from build123d import *

# Parameters (mm, degrees)
CYLINDER002_R     = 2.5
CYLINDER002_DEPTH = 18
CYLINDER003_R     = 4.5
CYLINDER003_DEPTH = 5
CYLINDER_R        = 2.5
CYLINDER_DEPTH    = 18
CYLINDER001_R     = 4.5
CYLINDER001_DEPTH = 5
PAD_DEPTH         = 12


with BuildPart() as cilindro002:
    # Cylinder002 → Cylinder002 (new body)
    with BuildSketch(Plane.XY):
        Circle(CYLINDER002_R)
    extrude(amount=CYLINDER002_DEPTH)


with BuildPart() as obj1:
    # Cylinder003 → Cylinder003 (new body)
    with BuildSketch(Plane.XY.offset(18)):
        Circle(CYLINDER003_R)
    extrude(amount=CYLINDER003_DEPTH)

    # Fusion001: union Cilindro002
    add(cilindro002.part)


with BuildPart() as obj1_1:
    # Fusion001 placement: moved
    add(obj1.part.moved(Location((58.5, 6, 0))))


with BuildPart() as cilindro:
    # Cylinder → Cylinder (new body)
    with BuildSketch(Plane.XY):
        Circle(CYLINDER_R)
    extrude(amount=CYLINDER_DEPTH)


with BuildPart() as tornillos:
    # Cylinder001 → Cylinder001 (new body)
    with BuildSketch(Plane.XY.offset(18)):
        Circle(CYLINDER001_R)
    extrude(amount=CYLINDER001_DEPTH)

    # Fusion: union Cilindro
    add(cilindro.part)


with BuildPart() as tornillos_1:
    # Fusion placement: moved
    add(tornillos.part.moved(Location((6.5, 6, 0))))

    # Fusion002: union obj1
    add(obj1_1.part)


with BuildPart() as obj2:
    # Sketch → Pad (new body)
    with BuildSketch(Plane.XZ):
        with BuildLine():
            Line((0, 0), (0, 11.5))
            Line((0, 11.5), (12.627017, 11.5))
            ThreePointArc((12.627017, 11.5), (20.5, 12.5), (12.627017, 13.5))
            Line((0, 13.5), (12.627017, 13.5))
            Line((0, 13.5), (0, 23))
            Line((0, 23), (65, 23))
            Line((65, 23), (65, 13.5))
            Line((65, 13.5), (52.372983, 13.5))
            ThreePointArc((52.372983, 13.5), (44.5, 12.5), (52.372983, 11.5))
            Line((65, 11.5), (52.372983, 11.5))
            Line((65, 0), (65, 11.5))
            Line((0, 0), (65, 0))
        make_face()
    extrude(amount=-PAD_DEPTH)

    # Cut: cut Tornillos
    add(tornillos_1.part, mode=Mode.SUBTRACT)


solid = obj2.part
Read the model definition and answer for the solid it produces. Units are mm, in the model's axes. A direction names the side the tool comes from. Coordinates: 2 decimals unless noted, no trailing zeros. Write each loop counter-clockwise with the first axis right and the second up, starting at its lowest first coordinate (ties: lowest second). Pieces come first, ordered by that corner, then holes. Notation, with made-up numbers: M 37.25,70 L 49.25,70 A8 ccw 49.25,79 Z; hole C 2,77 d11. An arc over 180 degrees is marked long. Use a Markdown table: item, result.
Q1. Which of the six approach directions +Z, -Z, +X, -X, +Y, -Y give full straight-line access (tool end or side, diameter ignored) to faces 1 (the face through (6, 3, 13.5)), 2 (the face through (8.885, 6.751, 15.718)), 3 (the face through (8.4, 4.1, 18))?
Answer block:
| item | result |
|---|---|
| face 1 | -X, +Y, -Y |
| face 2 | +Z, -Z |
| face 3 | +Z |
Q2. The part is cut by section B-B, the plane z = 9.5. Write down the section's boundary in (x, y), then the cut area to 3 significant figures.
Answer block:
| item | result |
|---|---|
| outline | M 0,0 L 13.85,0 L 13.85,12 L 0,12 Z; M 19.15,0 L 45.85,0 L 45.85,12 L 19.15,12 Z; M 51.15,0 L 65,0 L 65,12 L 51.15,12 Z; hole C 6.5,6 d5; hole C 58.5,6 d5 |
| area | 614 mm2 |
Q3. Determine the mould class of faces 4 (the face through (59, 3, 11.5)), 5 (the face through (0, 6, 18)), 6 (the face through (59, 3, 13.5)), 7 (the face through (32, 6, 0)) for opening direction Z: released by +Z, released by -Z, zero draft, split by the parting line, or undercut.
Answer block:
| item | result |
|---|---|
| face 4 | undercut |
| face 5 | zero draft |
| face 6 | undercut |
| face 7 | released by -Z |
Q4. Straight lines are drawn through the part: L1, parallel to X at y = 6, z = 5.25; L2, parallel to Z at x = 55, y = 1; L3, parallel to Y at x = 58.5, z = 20.65. For each, find the intervals that lie inside material, in ascending order. Write a range as [from, to].
Answer block:
| item | result |
|---|---|
| L1 | x = [0, 4], [9, 56], [61, 65] |
| L2 | z = [0, 11.5], [13.5, 23] |
| L3 | y = [0, 1.5], [10.5, 12] |
Q5. The part is cut by section C-C, the plane x = 6.5. Write down the section's boundary in (y, z), then the cut area to 3 significant figures.
Answer block:
| item | result |
|---|---|
| outline | M 0,0 L 3.5,0 L 3.5,11.5 L 0,11.5 Z; M 0,13.5 L 3.5,13.5 L 3.5,18 L 1.5,18 L 1.5,23 L 0,23 Z; M 8.5,0 L 12,0 L 12,11.5 L 8.5,11.5 Z; M 8.5,13.5 L 12,13.5 L 12,23 L 10.5,23 L 10.5,18 L 8.5,18 Z |
| area | 127 mm2 |
Q6. The part is cut by section A-A, the plane x = 48.5. Write down the section's boundary in (y, z).
Answer block:
| item | result |
|---|---|
| outline | M 0,0 L 12,0 L 12,8.5 L 0,8.5 Z; M 0,16.5 L 12,16.5 L 12,23 L 0,23 Z |
Q7. The part is cut by section D-D, the plane z = 21.75. Write down the section's boundary in (x, y).
Answer block:
| item | result |
|---|---|
| outline | M 0,0 L 65,0 L 65,12 L 0,12 Z; hole C 6.5,6 d9; hole C 58.5,6 d9 |
